```python
from build123d import *

# Parameters (mm, degrees)
SKETCH1_W           = 78
SKETCH1_H           = 15
SKETCH1_R           = 2.5
BOSS_EXTRUDE1_DEPTH = 3
SKETCH1_3_R         = 1.75
BOSS_EXTRUDE2_DEPTH = 0.5
FILLET1_R           = 0.7
BOSS_EXTRUDE3_START = -7
SKETCH2_R           = 2.5
BOSS_EXTRUDE3_DEPTH = 7


with BuildPart() as part:
    # Sketch1 → Boss-Extrude1 (new body)
    with BuildSketch(Plane(origin=(0, 0, 0), x_dir=(1, 0, 0), z_dir=(0, 1, 0))):
        with Locations((39, 7.5)):
            Rectangle(SKETCH1_W, SKETCH1_H)
        with Locations(Location((69, 7.5, 0), (0, 0, 270))):
            Circle(SKETCH1_R, mode=Mode.SUBTRACT)
        with Locations(Location((9, 7.5, 0), (0, 0, 270))):
            Circle(SKETCH1_R, mode=Mode.SUBTRACT)
        Polygon((46.636751, 10), (45.193376, 12.5), (42.306624, 12.5), (40.863249, 10), (42.306624, 7.5), (45.193376, 7.5), align=None, mode=Mode.SUBTRACT)
        Polygon((35.693376, 12.5), (32.806624, 12.5), (31.363249, 10), (32.806624, 7.5), (35.693376, 7.5), (37.136751, 10), align=None, mode=Mode.SUBTRACT)
    extrude(amount=BOSS_EXTRUDE1_DEPTH)

    # Sketch1_3 → Boss-Extrude2 (add)
    # profile 1 of 2: a face of its own
    with BuildSketch(Plane(origin=(0, 0, 0), x_dir=(1, 0, 0), z_dir=(0, 1, 0))):
        Polygon((37.136751, 10), (35.693376, 12.5), (32.806624, 12.5), (31.363249, 10), (32.806624, 7.5), (35.693376, 7.5), align=None)
        with Locations(Location((34.25, 10, 0), (0, 0, 270))):
            Circle(SKETCH1_3_R, mode=Mode.SUBTRACT)
    # profile 2 of 2: a face of its own
    with BuildSketch(Plane(origin=(0, 0, 0), x_dir=(1, 0, 0), z_dir=(0, 1, 0))):
        Polygon((45.193376, 7.5), (46.636751, 10), (45.193376, 12.5), (42.306624, 12.5), (40.863249, 10), (42.306624, 7.5), align=None)
        with Locations(Location((43.75, 10, 0), (0, 0, 270))):
            Circle(SKETCH1_3_R, mode=Mode.SUBTRACT)
    extrude(amount=BOSS_EXTRUDE2_DEPTH)

    # Fillet1
    fillet1_edges = [part.edges().sort_by_distance(p)[0] for p in [
        (0, 1.5, 0),
        (0, 1.5, -15),
        (78, 1.5, -15),
        (78, 1.5, 0),
    ]]
    fillet(fillet1_edges, radius=FILLET1_R)

    # Sketch2 → Boss-Extrude3 (add)
    # profile 1 of 2: a face of its own
    with BuildSketch(Plane(origin=(0, 0, 0), x_dir=(-1, 0, 0), z_dir=(0, -1, 0)).offset(BOSS_EXTRUDE3_START)):
        with BuildLine():
            Line((-77.3, 0), (-60, 0))
            Line((-60, 0), (-60, 15))
            Line((-60, 15), (-77.3, 15))
            ThreePointArc((-77.3, 15), (-77.794975, 14.794975), (-78, 14.3))
            Line((-78, 14.3), (-78, 0.7))
            ThreePointArc((-78, 0.7), (-77.794975, 0.205025), (-77.3, 0))
        make_face()
        with Locations(Location((-69, 7.5, 0), (0, 0, 90))):
            Circle(SKETCH2_R, mode=Mode.SUBTRACT)
    # profile 2 of 2: a face of its own
    with BuildSketch(Plane(origin=(0, 0, 0), x_dir=(-1, 0, 0), z_dir=(0, -1, 0)).offset(BOSS_EXTRUDE3_START)):
        with BuildLine():
            Line((-18, 15), (-18, 0))
            Line((-18, 0), (-0.7, 0))
            ThreePointArc((-0.7, 0), (-0.205025, 0.205025), (0, 0.7))
            Line((0, 0.7), (0, 14.3))
            ThreePointArc((0, 14.3), (-0.205025, 14.794975), (-0.7, 15))
            Line((-0.7, 15), (-18, 15))
        make_face()
        with Locations(Location((-9, 7.5, 0), (0, 0, 90))):
            Circle(SKETCH2_R, mode=Mode.SUBTRACT)
    extrude(amount=BOSS_EXTRUDE3_DEPTH)


solid = part.part
```
Design review of the part built by this model. Coordinates are the model's own, in mm. A direction names the side the tool comes from. Coordinates: 2 decimals unless noted, no trailing zeros. Loops run counter-clockwise (first coordinate to the right, second up) from the corner with the lowest first, then second, coordinate; pieces in that order, holes last. Notation, with made-up numbers: (76, -13.5) -> (115, -13.5) arc R11 cw to (115, -8.5) -> close; hole circle Ø6 at (83.5, 13.25). An arc over 180 degrees is marked (long way). Answer as a JSON object with one key per item and string values.
Q1. The part is to be moulded in two halves that separate along X. For faces 1 (the flat face through (78, 4, -8)), 2 (the flat face through (32.095, 1.732, -11.268)), 3 (the flat face through (39.5, 2.8, 0)), say which applies: +X half, -X half, draft (parallel to the pull), parting line (faces both ways), or undercut.
Answer block:
{"face 1": "+X half", "face 2": "undercut", "face 3": "draft"}
Q2. Clearance check with flat-ended pins moving along their axes: pin 1 Ø5.5 at (x, z) = (33.5, -9) entering from +Y; pin 2 Ø1.5 at (x, z) = (43.5, -9.5) entering from +Y. State where each tip first meets the part, or that it passes through.
Answer block:
{"pin 1": "stops at y = 3", "pin 2": "passes through"}
Q3. Take a section at A-A on y = 5.75. Give the boundary of the cut face in (x, z), plus the area to 3 significant figures.
Answer block:
{"outline": "(0, -14.3) arc R0.7 ccw to (0.7, -15) -> (18, -15) -> (18, 0) -> (0.7, 0) arc R0.7 ccw to (0, -0.7) -> close; (60, -15) -> (77.3, -15) arc R0.7 ccw to (78, -14.3) -> (78, -0.7) arc R0.7 ccw to (77.3, 0) -> (60, 0) -> close; hole circle Ø5 at (9, -7.5); hole circle Ø5 at (69, -7.5)", "area": "500 mm^2"}
Q4. To check wall thickness, follow L1, parallel to X at y = 1, z = -11.75; L2, parallel to X at y = 3.75, z = -9; L3, parallel to X at y = 4.25, z = -5.25. State the ranges of each line that lie inside material, in increasing order.
Answer block:
{"L1": "x = 0 to 32.37, 36.13 to 41.87, 45.63 to 78", "L2": "x = 0 to 7, 11 to 18, 60 to 67, 71 to 78", "L3": "x = 0 to 7.91, 10.09 to 18, 60 to 67.91, 70.09 to 78"}
Q5. Take a section at B-B on x = 43.75. Give the boundary of the cut face in (y, z), plus the area to 4 significant figures.
Answer block:
{"outline": "(0, -15) -> (3, -15) -> (3, -12.5) -> (0.5, -12.5) -> (0.5, -11.75) -> (0, -11.75) -> close; (0, -8.25) -> (0.5, -8.25) -> (0.5, -7.5) -> (3, -7.5) -> (3, 0) -> (0, 0) -> close", "area": "30.75 mm^2"}
Q6. Tool access review of faces 4 (the flat face through (36.425, 1.732, -11.232)), 5 (the flat face through (0, 4, -7)), 6 (the flat face through (39, 3, -8)): name each direction out of +Z, -Z, +X, -X, +Y, -Y from which nothing blocks a thin tool from reaching the whole face with its end or side.
Answer block:
{"face 4": "+Y", "face 5": "+Z, -Z, -X, +Y, -Y", "face 6": "+Z, -Z, +Y"}
Q7. Take a section at C-C on z = -2.25. Give the boundary of the cut face in (x, y).
Answer block:
{"outline": "(0, 0) -> (78, 0) -> (78, 7) -> (60, 7) -> (60, 3) -> (18, 3) -> (18, 7) -> (0, 7) -> close"}
Q8. Take a section at D-D on y = 2.25. Give the boundary of the cut face in (x, z).
Answer block:
{"outline": "(0, -14.3) arc R0.7 ccw to (0.7, -15) -> (77.3, -15) arc R0.7 ccw to (78, -14.3) -> (78, -0.7) arc R0.7 ccw to (77.3, 0) -> (0.7, 0) arc R0.7 ccw to (0, -0.7) -> close; hole circle Ø5 at (9, -7.5); hole (31.36, -10) -> (32.81, -12.5) -> (35.69, -12.5) -> (37.14, -10) -> (35.69, -7.5) -> (32.81, -7.5) -> close; hole (40.86, -10) -> (42.31, -12.5) -> (45.19, -12.5) -> (46.64, -10) -> (45.19, -7.5) -> (42.31, -7.5) -> close; hole circle Ø5 at (69, -7.5)"}
